from build123d import *

# Parameters (mm, degrees)
BOSS_EXTRUDE1_DEPTH = 5
FILLET1_R           = 5
FILLET3_R           = 1
FILLET4_R           = 1


with BuildPart() as part:
    # Sketch1 → Boss-Extrude1 (new body)
    with BuildSketch(Plane.XY):
        Polygon((0, 5), (0, 19.982808697), (0, 25), (10, 25), (10, 21.6), (5, 21.6), (5, 20), (20, 20), (20, 5), (20, 0), (15, 0), (15, 5), (11.5, 5), (11.5, 8), (12.6, 8), (12.6, 10.3), (11.5, 10.3), (11.5, 15), (8.5, 15), (8.5, 10.3), (7.4, 10.3), (7.4, 8), (8.5, 8), (8.5, 5), (5, 5), (5, 0), (0, 0), align=None)
    extrude(amount=BOSS_EXTRUDE1_DEPTH)

    # Fillet1
    fillet1_edges = [part.edges().sort_by_distance(p)[0] for p in [
        (0, 25, 2.5),
    ]]
    fillet(fillet1_edges, radius=FILLET1_R)

    # Fillet3
    fillet3_edges = [part.edges().sort_by_distance(p)[0] for p in [
        (10, 21.6, 2.5),
        (20, 20, 2.5),
    ]]
    fillet(fillet3_edges, radius=FILLET3_R)

    # Fillet4
    fillet4_edges = [part.edges().sort_by_distance(p)[0] for p in [
        (10, 25, 2.5),
    ]]
    fillet(fillet4_edges, radius=FILLET4_R)


solid = part.part
Source: CAD feature listing. Evaluate the final solid. Frame: model axes, mm. A direction names the side the tool comes from. Round coordinates to 2 decimals unless told otherwise and drop trailing zeros. Write each loop counter-clockwise with the first axis right and the second up, starting at its lowest first coordinate (ties: lowest second). Pieces come first, ordered by that corner, then holes. Notation, with made-up numbers: M 55.25,52.5 L 68.25,52.5 A29 ccw 68.25,76.5 Z; hole C -19.75,-1 d11. An arc over 180 degrees is marked long. One line per item, written item: value. Start each with the question number.
Item 1: Section query A-A (x = 8). Return the cut outline in (y, z).
Item 2: Section query C-C (z = 4.45). Return the cut outline in (x, y), plus the area to 3 significant figures.
Item 3: Mould query, pull axis Y, two halves, no side actions, for faces 1 (the flat face through (7.4, 9, 2)), 2 (the flat face through (5, 3, 2)), 3 (the flat face through (13, 5, 2)), 4 (the flat face through (7, 25, 2)). Classes: pulls with the +Y half, pulls with the -Y half, needs draft (parallel to the pull), parting line crosses it, or undercut.
Item 4: Ray query, L1, parallel to X at y = 3, z = 4.4; L2, parallel to X at y = 13.25, z = 3.7; L3, parallel to Y at x = 6, z = 3.95. Return the intervals inside material, ascending. Write a range as from..to.
Item 5: Pin query (flat end, axial travel): pin 1 (1 mm diameter, centred on x = 7.5, z = 3.5, fed in from -Y); pin 2 (0.8 mm diameter, centred on y = 20.5, z = 3, fed in from +X); pin 3 (1.2 mm diameter, centred on x = 12, z = 1.5, fed in from +Y). Return the tip coordinate at first contact, or that it passes through.
Item 6: Set-up query: faces 5 (the flat face through (8, 13, 0)), 6 (the flat face through (10, 23, 2)), 7 (the flat face through (12.6, 9, 2)), 8 (the flat face through (12, 20, 2)), 9 (the flat face through (8.5, 13, 2)). Return all of +Z, -Z, +X, -X, +Y, -Y with unobstructed straight access to the full face (end or side cutting, diameter ignored); none if empty.
Item 7: Section query B-B (y = 11). Return the cut outline in (x, z), plus the area to 3 significant figures.
Item 8: Section query D-D (x = 16). Return the cut outline in (y, z).
Result set:
1. outline: M 5,0 L 8,0 L 8,5 L 5,5 Z; M 10.3,0 L 20,0 L 20,5 L 10.3,5 Z; M 21.6,0 L 25,0 L 25,5 L 21.6,5 Z
2. outline: M 0,0 L 5,0 L 5,5 L 8.5,5 L 8.5,8 L 7.4,8 L 7.4,10.3 L 8.5,10.3 L 8.5,15 L 11.5,15 L 11.5,10.3 L 12.6,10.3 L 12.6,8 L 11.5,8 L 11.5,5 L 15,5 L 15,0 L 20,0 L 20,19 A1 ccw 19,20 L 5,20 L 5,21.6 L 9,21.6 A1 ccw 10,22.6 L 10,24 A1 ccw 9,25 L 5,25 A5 ccw 0,20 Z
2. area: 351 mm²
3. face 1: undercut
3. face 2: needs draft
3. face 3: pulls with the -Y half
3. face 4: pulls with the +Y half
4. L1: x = 0..5, 15..20
4. L2: x = 0..8.5, 11.5..20
4. L3: y = 5..20, 21.6..25
5. pin 1: stops at y = 5
5. pin 2: stops at x = 5
5. pin 3: stops at y = 20
6. face 5: -Z, +X, -X, +Y, -Y
6. face 6: +Z, -Z, +X, +Y
6. face 7: +Z, -Z
6. face 8: +Z, -Z, +X
6. face 9: +Z, -Z, -Y
7. outline: M 0,0 L 8.5,0 L 8.5,5 L 0,5 Z; M 11.5,0 L 20,0 L 20,5 L 11.5,5 Z
7. area: 85.0 mm²
8. outline: M 0,0 L 20,0 L 20,5 L 0,5 Z
